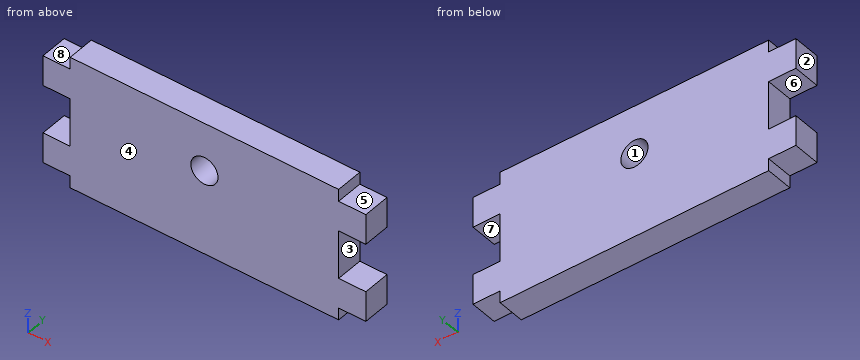
from build123d import *

# Parameters (mm, degrees)
BOSS_EXTRUDE1_DEPTH = 4.5
SKETCH2_R           = 2.25
CUT_EXTRUDE1_DEPTH  = 5.5


with BuildPart() as part:
    # Sketch1 → Boss-Extrude1 (new body)
    with BuildSketch(Plane(origin=(0, 0, 0), x_dir=(1, 0, 0), z_dir=(0, 1, 0))):
        Polygon((-22.225, -9), (-22.225, -11), (0, -11), (0, 11), (-22.225, 11), (-22.225, 9), (-26.725, 9), (-26.725, 4), (-22.225, 4), (-22.225, -4), (-26.725, -4), (-26.725, -9), align=None)
    boss_extrude1 = extrude(amount=BOSS_EXTRUDE1_DEPTH)

    # Mirror1: Boss-Extrude1 across plane
    add(boss_extrude1.mirror(Plane(origin=(0, 4.5, -11), x_dir=(0, 0, 1), z_dir=(-1, 0, 0))))

    # Sketch2 → Cut-Extrude1 (cut, through all)
    with BuildSketch(Plane(origin=(0, 4.5, 0), x_dir=(1, 0, 0), z_dir=(0, 1, 0))):
        with Locations((0, -3)):
            Circle(SKETCH2_R)
    extrude(amount=-CUT_EXTRUDE1_DEPTH, mode=Mode.SUBTRACT)


solid = part.part
Read the model definition and answer for the solid it produces. Units are mm, in the model's axes. Face numbers are marked on the shaded views. A direction names the side the tool comes from. Give positions to 0.01 mm unless a question says otherwise; leave off trailing zeros. Write each loop counter-clockwise with the first axis right and the second up, starting at its lowest first coordinate (ties: lowest second). Pieces come first, ordered by that corner, then holes. Notation, with made-up numbers: (3, -5) - (26, -5) arc R14 ccw to (26, 0) - close; hole circle Ø2 at (73, -3). An arc over 180 degrees is marked (long way). Use CSV: the item, a comma, the result in double quotes. Start each with the question number.
Item 1: Flat-ended cylindrical pins translate along their axes: P1, Ø1.6, axis at y = 2, z = 10, coming from the +X side (3 decimals); P2, Ø1.3, axis at x = -24.5, y = 2, coming from the -Z side; P3, Ø2, axis at x = 24.5, y = 2, coming from the +Z side. Find the tip coordinate at first contact, or state that the pin passes through.
Item 2: For the marked faces 5, 6, 7 and 8, determine the directions among +Z, -Z, +X, -X, +Y, -Y from which every point of the face is accessible in a straight line to the end or side of a thin tool.
Item 3: The mould has two halves that part along X. Classify the marked faces 1, 2, 3 and 4: pulls with the +X half, pulls with the -X half, needs draft (parallel to the pull), parting line crosses it, or undercut.
Item 4: The part is cut by section C-C, the plane y = 1.3. Give the vertices of the cut face in (x, z) (3 decimals).
Item 5: The part is cut by section D-D, the plane z = -9.5. Give the vertices of the cut face in (x, y) (3 decimals).
Item 6: The part is cut by section A-A, the plane x = 0. Give the vertices of the cut face in (y, z), and give its area (4 significant figures).
Item 7: Consider line 1 (Z direction, x = 0, y = 1); line 2 (X direction, y = 1.7, z = 3) (3 decimals); line 3 (X direction, y = 0.7, z = -3.5) (3 decimals). Determine where each line is inside the solid, lowest interval first.
Item 8: The part is cut by section B-B, the plane z = 3. Give the vertices of the cut face in (x, y) (3 decimals).
Taken from the geometry:
1,P1,"x = 22.225"
1,P2,"z = -9"
1,P3,"z = 9"
2,face 5,"+Z, +X, +Y, -Y"
2,face 6,"-X, +Y, -Y"
2,face 7,"+X, +Y, -Y"
2,face 8,"+Z, -X, +Y, -Y"
3,face 1,"undercut"
3,face 2,"pulls with the -X half"
3,face 3,"pulls with the +X half"
3,face 4,"needs draft"
4,outline,"(-26.725, -9) - (-22.225, -9) - (-22.225, -11) - (22.225, -11) - (22.225, -9) - (26.725, -9) - (26.725, -4) - (22.225, -4) - (22.225, 4) - (26.725, 4) - (26.725, 9) - (22.225, 9) - (22.225, 11) - (-22.225, 11) - (-22.225, 9) - (-26.725, 9) - (-26.725, 4) - (-22.225, 4) - (-22.225, -4) - (-26.725, -4) - close; hole circle Ø4.5 at (0, 3)"
5,outline,"(-22.225, 0) - (22.225, 0) - (22.225, 4.5) - (-22.225, 4.5) - close"
6,outline,"(0, -11) - (4.5, -11) - (4.5, 0.75) - (0, 0.75) - close; (0, 5.25) - (4.5, 5.25) - (4.5, 11) - (0, 11) - close"
6,area,"78.75 mm2"
7,line 1,"-11 to 0.75, 5.25 to 11"
7,line 2,"-22.225 to -2.25, 2.25 to 22.225"
7,line 3,"-22.225 to 22.225"
8,outline,"(-22.225, 0) - (-2.25, 0) - (-2.25, 4.5) - (-22.225, 4.5) - close; (2.25, 0) - (22.225, 0) - (22.225, 4.5) - (2.25, 4.5) - close"
